Here's how the part is built. I have some questions about the finished solid (model axes, mm). A direction names the side the tool comes from. Give positions to 0.01 mm unless a question says otherwise; leave off trailing zeros. Write each loop counter-clockwise with the first axis right and the second up, starting at its lowest first coordinate (ties: lowest second). Pieces come first, ordered by that corner, then holes. Notation, with made-up numbers: (15.25, -11.75) -> (70.25, -11.75) arc R20 cw to (70.25, 18.25) -> close; hole circle Ø8 at (22.5, 40). An arc over 180 degrees is marked (long way). Answer as CSV lines item,"result". Start each with the question number.
Autodesk Inventor part; units mm, degrees
ref_plane "YZ Plane" through (0, 0, 0) normal (1, 0, 0) x (0, 1, 0)
ref_plane "XZ Plane" through (0, 0, 0) normal (0, 1, 0) x (-1, 0, 0)
ref_plane "XY Plane" through (0, 0, 0) normal (0, 0, 1) x (1, 0, 0)
sketch "Sketch1" plane through (0, 0, 0) normal (0, 1, 0) x (-1, 0, 0)
  line L0 (-25.4, -12.7) -> (25.4, -12.7)
  line L1 (25.4, -12.7) -> (25.4, 12.7)
  line L2 (25.4, 12.7) -> (-25.4, 12.7)
  line L3 (-25.4, 12.7) -> (-25.4, -12.7)
  line L4 (-25.4, -12.7) -> (25.4, 12.7) construction
  line L5 (25.4, -12.7) -> (-25.4, 12.7) construction
  line L6 (22.225, -9.525) -> (-22.225, -9.525)
  line L7 (-22.225, -9.525) -> (-22.225, 9.525)
  line L8 (-22.225, 9.525) -> (22.225, 9.525)
  line L9 (22.225, 9.525) -> (22.225, -9.525)
  line L10 (22.225, -9.525) -> (-22.225, 9.525) construction
  line L11 (-22.225, -9.525) -> (22.225, 9.525) construction
  point P0 (0, 0)
  dimension "d0" = 50.8
  dimension "d1" = 25.4
  dimension "d2" = 44.45
  dimension "d3" = 19.05
extrude "Extrusion1" add sketch "Sketch1" along normal blind 609.6
sketch "Sketch2" plane through (-25.4, 0, 12.7) normal (0, 0, 1) x (1, 0, 0)
  line L0 (0, 609.6) -> (25.4, 609.6)
  line L1 (25.4, 609.6) -> (25.4, 584.2)
  line L2 (25.4, 584.2) -> (0, 584.2)
  line L3 (0, 584.2) -> (0, 609.6)
  circle A0 centre (25.4, 584.2) radius 6.35
  point P0 (25.4, 0)
  dimension "d6" = 25.4
  dimension "d7" = 25.4
  dimension "d8" = 12.7
extrude "Extrusion2" cut sketch "Sketch2" against normal blind 609.6 contours A0 L2 L1 | L1 L2 A0
sketch "Sketch4" plane through (0, 0, 0) normal (0, -1, 0) x (1, 0, 0)
  line L0 (22.225, 9.525) -> (22.225, -9.525)
  line L1 (22.225, -9.525) -> (-22.225, -9.525)
  line L2 (-22.225, -9.525) -> (-22.225, 9.525)
  line L3 (-22.225, 9.525) -> (22.225, 9.525)
  line L4 (25.4, -12.7) -> (-25.4, -12.7)
  line L5 (25.4, 12.7) -> (25.4, -12.7)
  line L6 (-25.4, 12.7) -> (25.4, 12.7)
  line L7 (-25.4, -12.7) -> (-25.4, 12.7)
  point P0 (0, 0)
extrude "Extrusion4" add sketch "Sketch4" along normal blind 12.7
sketch "Sketch6" plane through (0, 609.6, 0) normal (0, 1, 0) x (1, 0, 0)
  line L0 (22.225, 9.525) -> (22.225, -9.525)
  line L1 (22.225, -9.525) -> (-22.225, -9.525)
  line L2 (-22.225, -9.525) -> (-22.225, 9.525)
  line L3 (-22.225, 9.525) -> (22.225, 9.525)
  line L4 (25.4, 12.7) -> (-25.4, 12.7)
  line L5 (-25.4, 12.7) -> (-25.4, -12.7)
  line L6 (-25.4, -12.7) -> (25.4, -12.7)
  line L7 (25.4, -12.7) -> (25.4, 12.7)
  point P0 (0, 0)
extrude "Extrusion6" add sketch "Sketch6" along normal blind 63.5
sketch "Sketch8" plane through (-25.4, -12.7, 12.7) normal (0, 0, 1) x (1, 0, 0)
  line L0 (50.8, 0) -> (50.8, 685.8)
  line L1 (0, 685.8) -> (50.8, 685.8)
  line L2 (25.4, 685.8) -> (25.4, 341.8078)
  line L3 (25.4, 685.8) -> (369.3922, 685.8) construction
  line L4 (25.4, 341.8078) -> (25.4, 291.0078)
  circle A0 centre (25.4, 291.0078) radius 3.175
  circle A1 centre (25.4, 341.8078) radius 3.175
  point P0 (25.4, 12.7)
  dimension "d49" = 343.9922
  dimension "d50" = 90
  dimension "d51" = 50.8
  dimension "d52" = 180
  dimension "d53" = 6.35
  dimension "d54" = 6.35
extrude "Extrusion9" cut sketch "Sketch8" against normal blind 50.8
sketch "Sketch9" plane through (25.4, -12.7, 12.7) normal (1, 0, 0) x (0, 0, -1)
  line L0 (25.4, 0) -> (0, 0)
  line L1 (12.7, 0) -> (12.7, 84.1502)
  line L2 (12.7, 84.1502) -> (12.7, 46.0502)
  line L3 (12.7, 84.1502) -> (50.8, 84.1502) construction
  point P0 (12.7, 12.7)
  dimension "d57" = 84.1502
  dimension "d58" = 38.1
  dimension "d59" = 90
hole "Hole1" at (25.4, 71.4502, 0) at (25.4, 33.3502, 0) direction (-1, 0, 0) diameter 6.35 end through all
sketch "Sketch10" plane through (-25.4, -12.7, -12.7) normal (-1, 0, 0) x (0, 0, 1)
  line L0 (25.4, 0) -> (25.4, 685.8)
  line L1 (0, 685.8) -> (25.4, 685.8)
  line L2 (12.7, 685.8) -> (12.7, 254)
  line L3 (12.7, 254) -> (12.7, 203.2)
  circle A0 centre (12.7, 254) radius 3.175
  circle A1 centre (12.7, 203.2) radius 3.175
  point P0 (12.7, 12.7)
  dimension "d67" = 431.8
  dimension "d68" = 50.8
  dimension "d69" = 180
  dimension "d70" = 6.35
  dimension "d71" = 6.35
extrude "Extrusion10" cut sketch "Sketch10" against normal blind 50.8
properties part number "SuperSuperStructure"
Item 1: I'm going to push a flat-ended pin straight in: pin 1 (4 mm diameter, centred on y = 33.35, z = 0, fed in from -X). Where does the tip first touch, or does it pass through?
Item 2: For faces 1 (the face through (0, 325, -9.525)), 2 (the face through (25.4, 325, 0)), which set-ups out of +Z, -Z, +X, -X, +Y, -Y let a thin tool reach every point of the face, with its end or its side?
Item 3: If we section it at B-B (x = 13): Please give me the cut outline in (y, z) (3 decimals).
Item 4: If I drill on line 1 (Y direction, x = 0, z = 10.35); line 2 (Z direction, x = -1, y = 196.5) (3 decimals); line 3 (Z direction, x = 24, y = 190), over which ranges is the centre line in solid material (lowest first)? Write a range as [from, to].
Item 5: If we section it at A-A (y = 584.2): Please give me the cut outline in (x, z) (3 decimals), and give its area (3 significant figures).
Item 6: If we section it at C-C (y = 382.5): Please give me the cut outline in (x, z) (3 decimals).
Item 7: We'd pull the mould along Z, two halves only. Please class faces 3 (the face through (0, -12.7, 10)), 4 (the face through (-22.225, 325, 0)), 5 (the face through (0, 325, 12.7)): released by +Z, released by -Z, zero draft, split by the parting line, or undercut.
Final values:
1,pin 1,"through"
2,face 1,"+Y, -Y"
2,face 2,"+Z, -Z, +X, +Y, -Y"
3,outline,"(-12.7, -12.7) -> (673.1, -12.7) -> (673.1, -9.525) -> (-12.7, -9.525) -> close; (-12.7, 9.525) -> (673.1, 9.525) -> (673.1, 12.7) -> (-12.7, 12.7) -> close"
4,line 1,"[-12.7, 275.13], [281.48, 325.93], [332.28, 577.85], [590.55, 673.1]"
4,line 2,"[-12.7, -9.525], [9.525, 12.7]"
4,line 3,"[-12.7, -3.14], [3.14, 12.7]"
5,outline,"(-25.4, -12.7) -> (-6.35, -12.7) -> (-6.35, -9.525) -> (-22.225, -9.525) -> (-22.225, 9.525) -> (-6.35, 9.525) -> (-6.35, 12.7) -> (-25.4, 12.7) -> close; (6.35, -12.7) -> (25.4, -12.7) -> (25.4, 12.7) -> (6.35, 12.7) -> (6.35, 9.525) -> (22.225, 9.525) -> (22.225, -9.525) -> (6.35, -9.525) -> close"
5,area,"363 mm2"
6,outline,"(-25.4, -12.7) -> (25.4, -12.7) -> (25.4, 12.7) -> (-25.4, 12.7) -> close; hole (-22.225, -9.525) -> (22.225, -9.525) -> (22.225, 9.525) -> (-22.225, 9.525) -> close"
7,face 3,"zero draft"
7,face 4,"undercut"
7,face 5,"released by +Z"
